Part print with two shaded views. Sizes in mm from the minimum x, y, z corner. A direction names the side the tool comes from. Round coordinates to 2 decimals unless told otherwise and drop trailing zeros. Write each loop counter-clockwise with the first axis right and the second up, starting at its lowest first coordinate (ties: lowest second). Pieces come first, ordered by that corner, then holes. Notation, with made-up numbers: (12.5, 64) -> (30.5, 64) arc R25 cw to (30.5, 79) -> close; hole circle Ø5 at (56.5, 49). An arc over 180 degrees is marked (long way). Answer in a Markdown table with one row per item.
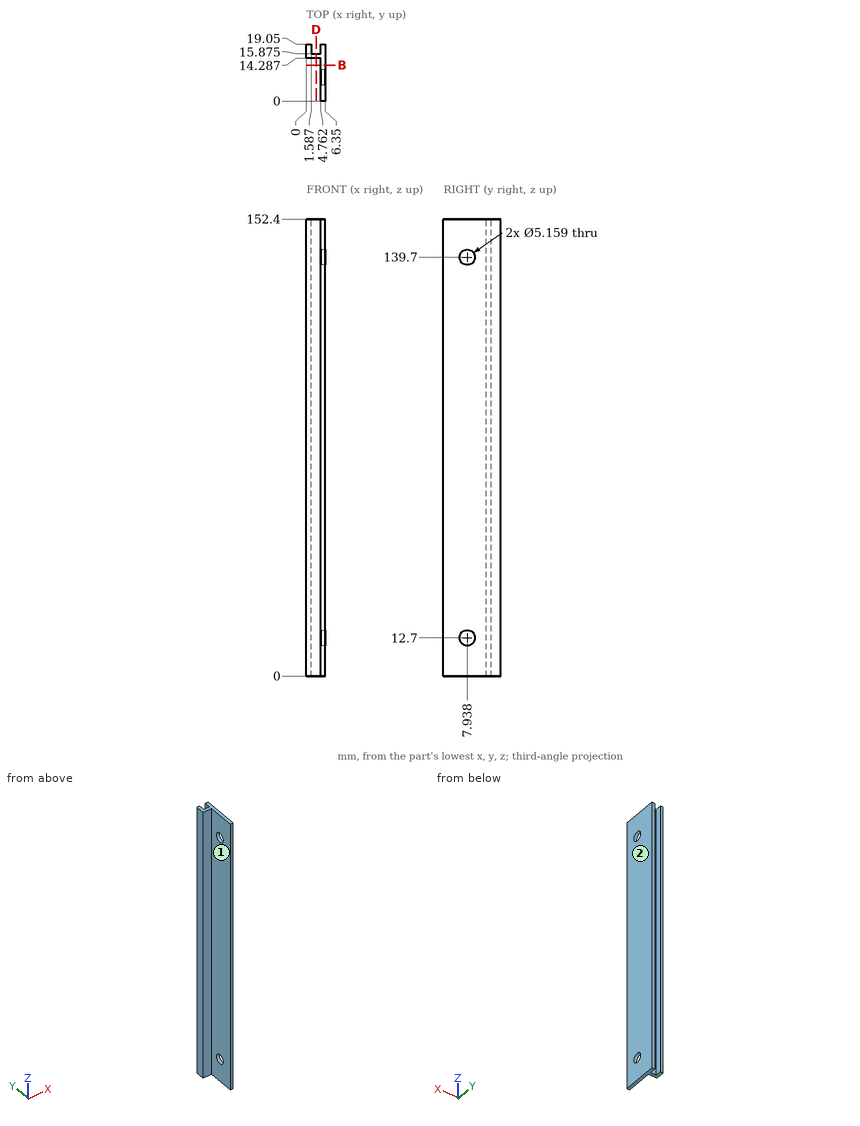
Q1. Wall check: line 1 (Y direction, x = 5.25, z = 12.7); line 2 (Z direction, x = 5, y = 8); line 3 (X direction, y = 17, z = 33). Give the ranges that are in metal, low to high. Write a range as [from, to].
A:
| item | result |
|---|---|
| line 1 | [0, 5.36], [10.52, 19.05] |
| line 2 | [0, 10.12], [15.28, 137.12], [142.28, 152.4] |
| line 3 | [0, 1.59], [4.76, 6.35] |
Q2. Saw through at B-B on y = 12. Write the cut outline in (x, z), plus the area to 3 significant figures.
A:
| item | result |
|---|---|
| outline | (4.76, 0) -> (6.35, 0) -> (6.35, 152.4) -> (4.76, 152.4) -> close |
| area | 242 mm² |
Q3. Saw through at D-D on x = 3.25. Write the cut outline in (y, z) (1 decimal).
A:
| item | result |
|---|---|
| outline | (14.3, 0) -> (15.9, 0) -> (15.9, 152.4) -> (14.3, 152.4) -> close |
Q4. Drop flat-ended pins along their axis: P1, Ø10, axis at y = 3, z = 25.5, coming from the -X side; P2, Ø2.5, axis at x = 1.5, z = 63.5, coming from the -Y side; P3, Ø1, axis at x = 2.5, z = 61.5, coming from the +Y side (1 decimal). Give the stop position or say it passes through.
A:
| item | result |
|---|---|
| P1 | x = 4.76 |
| P2 | y = 14.29 |
| P3 | y = 15.9 |
Q5. Which spindle directions (+Z, -Z, +X, -X, +Y, -Y) get a long thin tool onto all of the face, cutting with end or side? Do the marked faces 1 and 2. Say none if no direction does.
A:
| item | result |
|---|---|
| face 1 | +Z, -Z, -X, -Y |
| face 2 | +Z, -Z, +X, +Y, -Y |
